Part model, mm, in its own coordinate system. Face numbers are marked on the shaded views. A direction names the side the tool comes from. Coordinates: 2 decimals unless noted, no trailing zeros. Write each loop counter-clockwise with the first axis right and the second up, starting at its lowest first coordinate (ties: lowest second). Pieces come first, ordered by that corner, then holes. Notation, with made-up numbers: (26, 31.25) -> (75, 31.25) arc R25 ccw to (75, 43.25) -> close; hole circle Ø4 at (-20, 5). An arc over 180 degrees is marked (long way). Write item = value, one per line. Start each with the question number.
Q1. Tool access for the marked faces 5 and 6: list every direction of +Z, -Z, +X, -X, +Y, -Y with a clear straight run to the whole face (end or side of a thin tool).
Q2. Band-saw the part on B-B, the plane z = 16. Give the number of separate pieces and of enclosed holes in the cut face, plus the area to 3 significant figures.
Q3. Band-saw the part on C-C, the plane y = 37. List the corners of the cut face in (x, z).
Q4. Pin check, flat tips, straight feed: P1, Ø20, axis at x = 27, z = 10, coming from the -Y side; P2, Ø9, axis at y = 31.5, z = 5, coming from the +X side; P3, Ø8, axis at y = -10, z = 27, coming from the +X side. Stop position of each tip, or through.
Q5. Pull direction X, two halves, no side cores. Call the marked faces 1, 2, 3 and 4: released by +X, released by -X, zero draft, split by the parting line, or undercut.
Q6. Band-saw the part on D-D, the plane z = 22. List the corners of the cut face in (x, y) (3 decimals).
Q7. Band-saw the part on A-A, the plane x = 0. List the corners of the cut face in (y, z) (3 decimals), plus the area to 3 significant figures.
Q8. Probe line 1 (X direction, y = 31, z = 13); line 2 (Y direction, x = 0, z = 26.25) (3 decimals); line 3 (X direction, y = 30, z = 3.5). List the from-to ranges inside material, lowest first.
from build123d import *

# Parameters (mm, degrees)
F0_R     = 47.25
F0_R_2   = 2
F1_DEPTH = 18
F2_R     = 16.875
F3_DEPTH = 20
F7_R     = 3.25
F8_DEPTH = 25
F9_DEPTH = 25


with BuildPart() as f1:
    # F0 (on Top) → F1 (new body)
    with BuildSketch(Plane.XY):
        Circle(F0_R)
        with BuildLine():
            ThreePointArc((3, 43.1458283036), (30.5823682863, 30.5823682863), (43.1458283036, 3))
            ThreePointArc((43.1458283036, 3), (43.2239492303, 1.5009040394), (43.25, 0))
            ThreePointArc((43.25, 0), (43.2239492303, -1.5009040394), (43.1458283036, -3))
            ThreePointArc((43.1458283036, -3), (30.5823682863, -30.5823682863), (3, -43.1458283036))
            ThreePointArc((3, -43.1458283036), (0, -43.25), (-3, -43.1458283036))
            ThreePointArc((-3, -43.1458283036), (-30.5823682863, -30.5823682863), (-43.1458283036, -3))
            ThreePointArc((-43.1458283036, -3), (-43.25, 0), (-43.1458283036, 3))
            ThreePointArc((-43.1458283036, 3), (-30.5823682863, 30.5823682863), (-3, 43.1458283036))
            ThreePointArc((-3, 43.1458283036), (0, 43.25), (3, 43.1458283036))
        make_face(mode=Mode.SUBTRACT)
        with BuildLine():
            Line((43.1458283036, 3), (19.6472803461, 3))
            ThreePointArc((19.6472803461, 3), (19.8179883172, 1.5043151466), (19.875, 0))
            ThreePointArc((19.875, 0), (19.8179883172, -1.5043151466), (19.6472803461, -3))
            Line((19.6472803461, -3), (43.1458283036, -3))
            ThreePointArc((43.1458283036, -3), (43.2239492303, -1.5009040394), (43.25, 0))
            ThreePointArc((43.25, 0), (43.2239492303, 1.5009040394), (43.1458283036, 3))
        make_face()
        with Locations((31.5, 0)):
            Circle(F0_R_2, mode=Mode.SUBTRACT)
        with BuildLine():
            ThreePointArc((-19.6472803461, -3), (-19.875, 0), (-19.6472803461, 3))
            Line((-19.6472803461, 3), (-43.1458283036, 3))
            ThreePointArc((-43.1458283036, 3), (-43.25, 0), (-43.1458283036, -3))
            Line((-43.1458283036, -3), (-19.6472803461, -3))
        make_face()
        with Locations((-31.5, 0)):
            Circle(F0_R_2, mode=Mode.SUBTRACT)
        with BuildLine():
            ThreePointArc((-3, 19.6472803461), (0, 19.875), (3, 19.6472803461))
            Line((3, 19.6472803461), (3, 43.1458283036))
            ThreePointArc((3, 43.1458283036), (0, 43.25), (-3, 43.1458283036))
            Line((-3, 43.1458283036), (-3, 19.6472803461))
        make_face()
        with Locations((0, 31.5)):
            Circle(F0_R_2, mode=Mode.SUBTRACT)
        with BuildLine():
            Line((3, -43.1458283036), (3, -19.6472803461))
            ThreePointArc((3, -19.6472803461), (0, -19.875), (-3, -19.6472803461))
            Line((-3, -19.6472803461), (-3, -43.1458283036))
            ThreePointArc((-3, -43.1458283036), (0, -43.25), (3, -43.1458283036))
        make_face()
        with Locations((0, -31.5)):
            Circle(F0_R_2, mode=Mode.SUBTRACT)
        with BuildLine():
            Line((-3, -19.6472803461), (-3, -16.6061923691))
            ThreePointArc((-3, -16.6061923691), (-11.9324269325, -11.9324269325), (-16.6061923691, -3))
            Line((-16.6061923691, -3), (-19.6472803461, -3))
            ThreePointArc((-19.6472803461, -3), (-14.0537472761, -14.0537472761), (-3, -19.6472803461))
        make_face()
        with BuildLine():
            Line((19.6472803461, -3), (16.6061923691, -3))
            ThreePointArc((16.6061923691, -3), (11.9324269325, -11.9324269325), (3, -16.6061923691))
            Line((3, -16.6061923691), (3, -19.6472803461))
            ThreePointArc((3, -19.6472803461), (14.0537472761, -14.0537472761), (19.6472803461, -3))
        make_face()
        with BuildLine():
            ThreePointArc((3, 16.6061923691), (11.9324269325, 11.9324269325), (16.6061923691, 3))
            Line((16.6061923691, 3), (19.6472803461, 3))
            ThreePointArc((19.6472803461, 3), (14.0537472761, 14.0537472761), (3, 19.6472803461))
            Line((3, 19.6472803461), (3, 16.6061923691))
        make_face()
        with BuildLine():
            ThreePointArc((-16.6061923691, 3), (-11.9324269325, 11.9324269325), (-3, 16.6061923691))
            Line((-3, 16.6061923691), (-3, 19.6472803461))
            ThreePointArc((-3, 19.6472803461), (-14.0537472761, 14.0537472761), (-19.6472803461, 3))
            Line((-19.6472803461, 3), (-16.6061923691, 3))
        make_face()
        with BuildLine():
            ThreePointArc((-3, 16.6061923691), (0, 16.875), (3, 16.6061923691))
            Line((3, 16.6061923691), (3, 19.6472803461))
            ThreePointArc((3, 19.6472803461), (0, 19.875), (-3, 19.6472803461))
            Line((-3, 19.6472803461), (-3, 16.6061923691))
        make_face()
        with BuildLine():
            ThreePointArc((16.6061923691, 3), (16.8076637465, 1.5060094241), (16.875, 0))
            ThreePointArc((16.875, 0), (16.8076637465, -1.5060094241), (16.6061923691, -3))
            Line((16.6061923691, -3), (19.6472803461, -3))
            ThreePointArc((19.6472803461, -3), (19.8179883172, -1.5043151466), (19.875, 0))
            ThreePointArc((19.875, 0), (19.8179883172, 1.5043151466), (19.6472803461, 3))
            Line((19.6472803461, 3), (16.6061923691, 3))
        make_face()
        with BuildLine():
            ThreePointArc((-16.6061923691, -3), (-16.875, 0), (-16.6061923691, 3))
            Line((-16.6061923691, 3), (-19.6472803461, 3))
            ThreePointArc((-19.6472803461, 3), (-19.875, 0), (-19.6472803461, -3))
            Line((-19.6472803461, -3), (-16.6061923691, -3))
        make_face()
        with BuildLine():
            Line((3, -19.6472803461), (3, -16.6061923691))
            ThreePointArc((3, -16.6061923691), (0, -16.875), (-3, -16.6061923691))
            Line((-3, -16.6061923691), (-3, -19.6472803461))
            ThreePointArc((-3, -19.6472803461), (0, -19.875), (3, -19.6472803461))
        make_face()
    extrude(amount=F1_DEPTH)

    # F2 (on face) → F3 (join)
    with BuildSketch(Plane.XY.offset(18)):
        with BuildLine():
            ThreePointArc((19.6472803461, -3), (19.8179883172, -1.5043151466), (19.875, 0))
            ThreePointArc((19.875, 0), (19.8179883172, 1.5043151466), (19.6472803461, 3))
            ThreePointArc((19.6472803461, 3), (14.0537472761, 14.0537472761), (3, 19.6472803461))
            ThreePointArc((3, 19.6472803461), (0, 19.875), (-3, 19.6472803461))
            ThreePointArc((-3, 19.6472803461), (-14.0537472761, 14.0537472761), (-19.6472803461, 3))
            ThreePointArc((-19.6472803461, 3), (-19.875, 0), (-19.6472803461, -3))
            ThreePointArc((-19.6472803461, -3), (-14.0537472761, -14.0537472761), (-3, -19.6472803461))
            ThreePointArc((-3, -19.6472803461), (0, -19.875), (3, -19.6472803461))
            ThreePointArc((3, -19.6472803461), (14.0537472761, -14.0537472761), (19.6472803461, -3))
        make_face()
        Circle(F2_R, mode=Mode.SUBTRACT)
    extrude(amount=F3_DEPTH)

    # F7 (on line) → F8 (cut)
    with BuildSketch(Plane(origin=(0, 0, 0), x_dir=(-0.7071067812, 0.7071067812, 0), z_dir=(0.7071067812, 0.7071067812, 0))):
        with Locations((0, 28)):
            Circle(F7_R)
    extrude(amount=-F8_DEPTH, mode=Mode.SUBTRACT)

    # F7 (on line) → F9 (cut)
    with BuildSketch(Plane(origin=(0, 0, 0), x_dir=(-0.7071067812, 0.7071067812, 0), z_dir=(0.7071067812, 0.7071067812, 0))):
        with Locations((0, 28)):
            Circle(F7_R)
    extrude(amount=F9_DEPTH, mode=Mode.SUBTRACT)


solid = f1.part
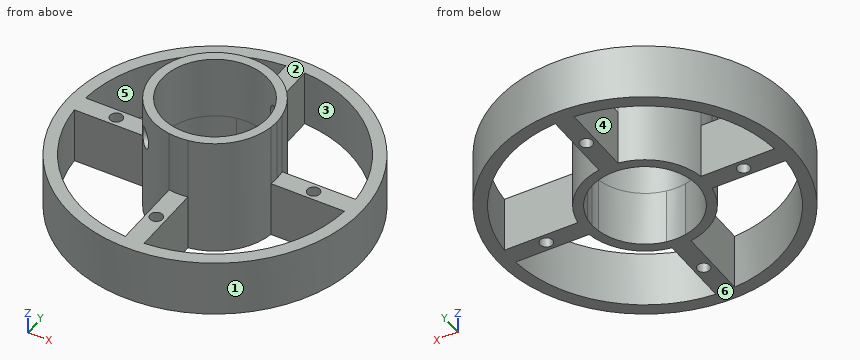
Ans:
q1.face_5 = +Z, -Z
q1.face_6 = -Z, +X, -X, +Y, -Y
q2.separate_pieces = 1
q2.enclosed_holes = 9
q2.area = 2,000 mm2
q3.outline = (-29.39, 0) -> (-22.4, 0) -> (-22.4, 18) -> (-29.39, 18) -> close; (-3, 0) -> (3, 0) -> (3, 18) -> (-3, 18) -> close; (22.4, 0) -> (29.39, 0) -> (29.39, 18) -> (22.4, 18) -> close
q4.P1 = -44.09
q4.P2 = 38.78
q4.P3 = 18.95
q5.face_1 = split by the parting line
q5.face_2 = zero draft
q5.face_3 = undercut
q5.face_4 = undercut
q6.outline = circle Ø39.75 at (0, 0); hole circle Ø33.75 at (0, 0)
q7.outline = (-47.25, 0) -> (-33.5, 0) -> (-33.5, 18) -> (-47.25, 18) -> close; (-29.5, 0) -> (-16.875, 0) -> (-16.875, 38) -> (-19.875, 38) -> (-19.875, 18) -> (-29.5, 18) -> close; (16.875, 0) -> (29.5, 0) -> (29.5, 18) -> (19.875, 18) -> (19.875, 38) -> (16.875, 38) -> close; (33.5, 0) -> (47.25, 0) -> (47.25, 18) -> (33.5, 18) -> close
q7.area = 1,070 mm2
q8.line_1 = -35.66 to -30.16, -3 to -1.94, 1.94 to 3, 30.16 to 35.66
q8.line_2 = -19.875 to -16.875, 16.875 to 19.875
q8.line_3 = -36.5 to -31.15, -3 to -1.32, 1.32 to 3, 31.15 to 36.5
